Part model, mm, in its own coordinate system. A direction names the side the tool comes from. Coordinates: 2 decimals unless noted, no trailing zeros. Write each loop counter-clockwise with the first axis right and the second up, starting at its lowest first coordinate (ties: lowest second). Pieces come first, ordered by that corner, then holes. Notation, with made-up numbers: M -26.5,7.5 L 6.5,7.5 A18 cw 6.5,17.5 Z; hole C 18.25,25 d11. An arc over 180 degrees is marked long. Use a Markdown table: item, result. Add a question column.
Q1. Wall check: L1, parallel to Z at x = -13, y = 2; L2, parallel to Z at x = -5, y = 8; L3, parallel to X at y = 9, z = 4.5. Give the ranges that are in metal, low to high. Write a range as from..to.
Q2. Slice it at A-A on x = -11. Write the cut outline in (y, z), then the cut area to 3 significant figures.
Q3. Slice it at C-C on z = -3.5. Write the cut outline in (x, y).
Q4. Pin check, flat tips, straight feed: pin 1 Ø1 at (x, z) = (10.5, -8.5) entering from +Y; pin 2 Ø3 at (y, z) = (6, 16) entering from +X; pin 3 Ø1 at (x, y) = (7.5, 1.5) entering from -Z; pin 4 Ø3 at (x, y) = (-14.5, 4) entering from +Z. Stop position of each tip, or through.
Q5. Slice it at D-D on x = -0.5. Write the cut outline in (y, z), then the cut area to 3 significant figures.
Q6. Mould opens along Z. For faces 1 (the flat face through (-18, 5, 0)), 2 (the flat face through (-12, 5, 13.8)), 3 (the flat face through (8, 5, -13.8)) say: released by +Z, released by -Z, zero draft, split by the parting line, or undercut.
Q7. Slice it at B-B on y = 1.5. Write the cut outline in (x, z), then the cut area to 3 significant figures.
Q8. Tool access for faces 4 (the flat face through (-6, 5, 16)), 5 (the flat face through (0, 5, -16)), 6 (the cylindrical face through (-16.521, 6.867, 4.771)), 7 (the flat face through (-4, 5, 10.2)), 8 (the flat face through (7, 5, 13.8)): list every direction of +Z, -Z, +X, -X, +Y, -Y with a clear straight run to the whole face (end or side of a thin tool).
from build123d import *

# Parameters (mm, degrees)
SKETCH1_W           = 29.2
SKETCH1_H           = 20.4
BOSS_EXTRUDE1_DEPTH = 9.6
SKETCH3_R           = 2.085
BOSS_EXTRUDE3_DEPTH = 3


with BuildPart() as part:
    # Sketch1 → Boss-Extrude1 (new body)
    with BuildSketch(Plane(origin=(0, 0, 0), x_dir=(1, 0, 0), z_dir=(0, 1, 0))):
        with BuildLine():
            Line((-6, 13.8), (-18, 13.8))
            ThreePointArc((-18, 13.8), (-24.5, 0), (-18, -13.8))
            Line((-18, -13.8), (-6, -13.8))
            Line((-6, -13.8), (-6, -17.8))
            Line((-6, -17.8), (0, -17.8))
            Line((0, -17.8), (0, -13.8))
            Line((0, -13.8), (15, -13.8))
            Line((15, -13.8), (15, 13.8))
            Line((15, 13.8), (0, 13.8))
            Line((0, 13.8), (0, 17.8))
            Line((0, 17.8), (-6, 17.8))
            Line((-6, 17.8), (-6, 13.8))
        make_face()
        with Locations((-3.4, 0)):
            Rectangle(SKETCH1_W, SKETCH1_H, mode=Mode.SUBTRACT)
    extrude(amount=BOSS_EXTRUDE1_DEPTH)

    # Sketch3 → Boss-Extrude3 (add)
    with BuildSketch(Plane(origin=(-18, 0, 0), x_dir=(0, 0, -1), z_dir=(1, 0, 0))):
        with Locations((-4.5, 4.8)):
            Circle(SKETCH3_R)
        with Locations((4.5, 4.8)):
            Circle(SKETCH3_R)
    extrude(amount=BOSS_EXTRUDE3_DEPTH)


solid = part.part
Recorded:
| question | item | result |
|---|---|---|
| 1 | L1 | -13.8..-10.2, 10.2..13.8 |
| 1 | L2 | -17.8..-10.2, 10.2..17.8 |
| 1 | L3 | -23.93..-18, 11.2..15 |
| 2 | outline | M 0,-13.8 L 9.6,-13.8 L 9.6,-10.2 L 0,-10.2 Z; M 0,10.2 L 9.6,10.2 L 9.6,13.8 L 0,13.8 Z |
| 2 | area | 69.1 mm² |
| 3 | outline | M -24.15,0 L -18,0 L -18,2.97 L -15,2.97 L -15,6.63 L -18,6.63 L -18,9.6 L -24.15,9.6 Z; M 11.2,0 L 15,0 L 15,9.6 L 11.2,9.6 Z |
| 4 | pin 1 | through |
| 4 | pin 2 | x = 0 |
| 4 | pin 3 | z = -13.8 |
| 4 | pin 4 | z = 13.8 |
| 5 | outline | M 0,-17.8 L 9.6,-17.8 L 9.6,-10.2 L 0,-10.2 Z; M 0,10.2 L 9.6,10.2 L 9.6,17.8 L 0,17.8 Z |
| 5 | area | 146 mm² |
| 6 | face 1 | undercut |
| 6 | face 2 | released by +Z |
| 6 | face 3 | released by -Z |
| 7 | outline | M -18,-13.8 L -6,-13.8 L -6,-17.8 L 0,-17.8 L 0,-13.8 L 15,-13.8 L 15,13.8 L 0,13.8 L 0,17.8 L -6,17.8 L -6,13.8 L -18,13.8 A17.9 ccw Z; hole M -18,-10.2 L 11.2,-10.2 L 11.2,10.2 L -18,10.2 Z |
| 7 | area | 488 mm² |
| 8 | face 4 | +Z, -X, +Y, -Y |
| 8 | face 5 | -Z, +X, +Y, -Y |
| 8 | face 6 | none |
| 8 | face 7 | +Y, -Y |
| 8 | face 8 | +Z, +X, +Y, -Y |
